```python
from build123d import *

# Parameters (mm, degrees)
SKETCH1_R           = 1.5
BOSS_EXTRUDE1_DEPTH = 3.05


with BuildPart() as part:
    # Sketch1 → Boss-Extrude1 (new body)
    with BuildSketch(Plane(origin=(0, 0, 0), x_dir=(1, 0, 0), z_dir=(0, 1, 0))):
        Polygon((3.05, 17), (3.05, 12), (0, 12), (0, 4), (3.05, 4), (3.05, 0), (63.05, 0), (63.05, 4), (66.1, 4), (66.1, 12), (63.05, 12), (63.05, 17), align=None)
        with Locations(Location((54.05, 7, 0), (0, 0, 270))):
            Circle(SKETCH1_R, mode=Mode.SUBTRACT)
        with Locations(Location((12.05, 7, 0), (0, 0, 270))):
            Circle(SKETCH1_R, mode=Mode.SUBTRACT)
    extrude(amount=BOSS_EXTRUDE1_DEPTH)

    # Sketch5 → CSK for M3 Flat Head Machine Screw1 (revolve, cut)
    with BuildSketch(Plane(origin=(12.05, 3.05, -7), x_dir=(0, 0, 1), z_dir=(1, 0, 0))):
        Polygon((0, 0), (0, 3.05), (1.5, 3.05), (1.5, 1.65), (3.15, 0), align=None)
    revolve(axis=Axis((12.05, 9.4, -7), (0, -1, 0)), mode=Mode.SUBTRACT)

    # Sketch7 → CSK for M3 Flat Head Machine Screw2 (revolve, cut)
    with BuildSketch(Plane(origin=(54.05, 3.05, -7), x_dir=(0, 0, 1), z_dir=(1, 0, 0))):
        Polygon((0, 0), (0, 3.05), (1.5, 3.05), (1.5, 1.65), (3.15, 0), align=None)
    revolve(axis=Axis((54.05, 9.4, -7), (0, -1, 0)), mode=Mode.SUBTRACT)


solid = part.part
```
Geometry check sheet. Reference: the model listing, model coordinates, mm. A direction names the side the tool comes from. Give positions to 0.01 mm unless a question says otherwise; leave off trailing zeros. Order: outer loops, then holes, each group sorted by start corner. A loop starts at its lowest first (then second) coordinate and runs counter-clockwise, first axis right, second up. Notation, with made-up numbers: (68, 69) - (106, 69) arc R5 ccw to (106, 75) - close; hole circle Ø11 at (63.5, -6). An arc over 180 degrees is marked (long way). Answer in a Markdown table with one row per item. Add a question column.
Q1. Cross-section at B-B, the plane z = -7. Enter the section's corners in (x, y), then the cut area to 3 significant figures.
Q2. Cross-section at C-C, the plane y = 0.8. Enter the section's corners in (x, z).
Q3. Material ranges on probe 1 along X at (y, z) = (0.3, -7); probe 2 along Z at (x, y) = (12.05, 0.4); probe 3 along X at (y, z) = (0.55, -15.5), recorded low to high. Write a range as from..to.
Q4. Cross-section at A-A, the plane x = 12.05. Enter the section's corners in (y, z).
Q5. Tool access check on faces 4 (the flat face through (63.05, 2, -14)), 5 (the flat face through (63.05, 2, -2)), 6 (the flat face through (3.05, 2, -15)). Record the directions out of +Z, -Z, +X, -X, +Y, -Y that give a thin tool (end or side, any length) a straight path to the whole face; none if there is none.
Q6. Cross-section at D-D, the plane z = -2.5. Enter the section's corners in (x, y), then the cut area to 3 significant figures.
Q7. Mould release check, pull along Z, two halves, no side actions. Record for faces 1 (the cylindrical face through (11.14, 0.69, -8.19)), 2 (the flat face through (33, 2, 0)), 3 (the flat face through (3.05, 2, -2)): pulls with the +Z half, pulls with the -Z half, needs draft (parallel to the pull), parting line crosses it, or undercut.
Q8. Gauge pin test, flat ends, axial feed: pin 1 (1.5 mm diameter, centred on y = 1, z = -14, fed in from +X); pin 2 (0.9 mm diameter, centred on y = 1, z = -2, fed in from -X); pin 3 (0.9 mm diameter, centred on x = 2, y = 1, fed in from +Z). Record the tip position at first contact, or that the pin passes through.
Check values:
| question | item | result |
|---|---|---|
| 1 | outline | (0, 0) - (10.55, 0) - (10.55, 1.4) - (8.9, 3.05) - (0, 3.05) - close; (13.55, 0) - (52.55, 0) - (52.55, 1.4) - (50.9, 3.05) - (15.2, 3.05) - (13.55, 1.4) - close; (55.55, 0) - (66.1, 0) - (66.1, 3.05) - (57.2, 3.05) - (55.55, 1.4) - close |
| 1 | area | 178 mm^2 |
| 2 | outline | (0, -12) - (3.05, -12) - (3.05, -17) - (63.05, -17) - (63.05, -12) - (66.1, -12) - (66.1, -4) - (63.05, -4) - (63.05, 0) - (3.05, 0) - (3.05, -4) - (0, -4) - close; hole circle Ø3 at (12.05, -7); hole circle Ø3 at (54.05, -7) |
| 3 | probe 1 | x = 0..10.55, 13.55..52.55, 55.55..66.1 |
| 3 | probe 2 | z = -17..-8.5, -5.5..0 |
| 3 | probe 3 | x = 3.05..63.05 |
| 4 | outline | (0, -17) - (3.05, -17) - (3.05, -10.15) - (1.4, -8.5) - (0, -8.5) - close; (0, -5.5) - (1.4, -5.5) - (3.05, -3.85) - (3.05, 0) - (0, 0) - close |
| 5 | face 4 | -Z, +X, +Y, -Y |
| 5 | face 5 | +Z, +X, +Y, -Y |
| 5 | face 6 | -Z, -X, +Y, -Y |
| 6 | outline | (3.05, 0) - (63.05, 0) - (63.05, 3.05) - (3.05, 3.05) - close |
| 6 | area | 183 mm^2 |
| 7 | face 1 | undercut |
| 7 | face 2 | pulls with the +Z half |
| 7 | face 3 | needs draft |
| 8 | pin 1 | stops at x = 63.05 |
| 8 | pin 2 | stops at x = 3.05 |
| 8 | pin 3 | stops at z = -4 |
